Design review of the part built by this model. Coordinates are the model's own, in mm. Face numbers are marked on the shaded views. A direction names the side the tool comes from. Give positions to 0.01 mm unless a question says otherwise; leave off trailing zeros. Order: outer loops, then holes, each group sorted by start corner. A loop starts at its lowest first (then second) coordinate and runs counter-clockwise, first axis right, second up.
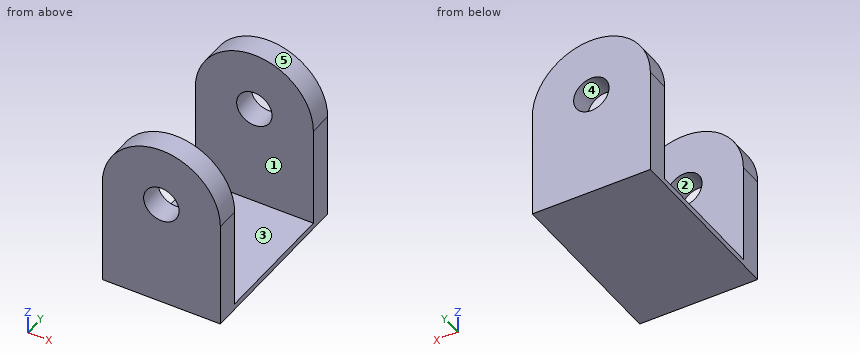
```python
from build123d import *

# Parameters (mm, degrees)
F0_R     = 15
F0_W     = 100
F0_H     = 5
F2_DEPTH = 150
F1_W     = 20
F1_H     = 200
F3_DEPTH = 116.7


with BuildPart() as f2:
    # F0 (on Front) → F2 (new body)
    with BuildSketch(Plane.XZ):
        with BuildLine():
            Line((0, 90), (0, 5))
            Line((0, 5), (100, 5))
            Line((100, 5), (100, 90))
            ThreePointArc((100, 90), (50, 140), (0, 90))
        make_face()
        with Locations((50, 90)):
            Circle(F0_R, mode=Mode.SUBTRACT)
        with Locations((50, 2.5)):
            Rectangle(F0_W, F0_H)
    extrude(amount=-F2_DEPTH)

    # F1 (on Right) → F3 (intersect)
    with BuildSketch(Plane.YZ):
        Polygon((0, 5), (0, 0), (150, 0), (150, 5), (130, 5), (20, 5), align=None)
        with Locations((10, 105)):
            Rectangle(F1_W, F1_H)
        with Locations((140, 105)):
            Rectangle(F1_W, F1_H)
    extrude(amount=F3_DEPTH, mode=Mode.INTERSECT)


solid = f2.part
```
1. Take a section at C-C (x = 31). State the section outline as (y, z) points, then the cut area to 3 significant figures.
Recorded:
outline: (0, 0) - (150, 0) - (150, 136.25) - (130, 136.25) - (130, 5) - (20, 5) - (20, 136.25) - (0, 136.25) - close
area: 6,000 mm2
2. Take a section at B-B (x = 50). State the section outline as (y, z) points, then the cut area to 3 significant figures.
Recorded:
outline: (0, 0) - (150, 0) - (150, 75) - (130, 75) - (130, 5) - (20, 5) - (20, 75) - (0, 75) - close; (0, 105) - (20, 105) - (20, 140) - (0, 140) - close; (130, 105) - (150, 105) - (150, 140) - (130, 140) - close
area: 4,950 mm2
3. Draft analysis for pull direction X (two halves, no side actions). For the marked faces 3, 4 and 5, state which applies: pulls with the +X half, pulls with the -X half, needs draft (parallel to the pull), parting line crosses it, or undercut.
Recorded:
face 3: needs draft
face 4: undercut
face 5: parting line crosses it
4. For line 1 along Y through (x, z) = (52, 15.5); line 2 along Z through (x, y) = (50, 141); line 3 along Z through (x, y) = (43, 44), list the stretches that pass through material, from the lowest coordinate up.
Recorded:
line 1: y = 0 to 20, 130 to 150
line 2: z = 0 to 75, 105 to 140
line 3: z = 0 to 5
5. Take a section at D-D (y = 108.5). State the section outline as (x, z) points.
Recorded:
outline: (0, 0) - (100, 0) - (100, 5) - (0, 5) - close
6. For pin 1 (12 mm diameter, centred on x = 31, z = 19.5, fed in from -Y), flat-tipped, find the tip position at first contact; note if it passes through.
Recorded:
pin 1: stops at y = 0
7. Machinability: for the marked faces 1 and 2, which of the approach directions +Z, -Z, +X, -X, +Y, -Y give a long, thin tool a straight path to every point of the face, cutting with its end or side? Answer none if there is none.
Recorded:
face 1: +Z, +X, -X
face 2: +Y, -Y
8. Take a section at A-A (z = 46.5). State the section outline as (x, y) points, then the cut area to 3 significant figures.
Recorded:
outline: (0, 0) - (100, 0) - (100, 20) - (0, 20) - close; (0, 130) - (100, 130) - (100, 150) - (0, 150) - close
area: 4,000 mm2
